Autodesk Inventor part; units mm, degrees
ref_plane "YZ Plane" through (0, 0, 0) normal (1, 0, 0) x (0, 1, 0)
ref_plane "XZ Plane" through (0, 0, 0) normal (0, 1, 0) x (-1, 0, 0)
ref_plane "XY Plane" through (0, 0, 0) normal (0, 0, 1) x (1, 0, 0)
sketch "스케치1" plane through (0, 0, 0) normal (0, 0, 1) x (1, 0, 0)
  line L0 (7.15, 10.1828) -> (7.15, 9)
  arc A0 (7.15, 9) -> (9.15, 7) centre (9.15, 9) ccw
  line L1 (9.15, 7) -> (11.2, 7)
  arc A1 (12.2, 6) -> (11.2, 7) centre (11.2, 6) ccw
  line L2 (12.2, 6) -> (12.2, -27)
  line L3 (-12.2, -27) -> (-12.2, 6)
  arc A2 (-11.2, 7) -> (-12.2, 6) centre (-11.2, 6) ccw
  line L4 (-11.2, 7) -> (-9.15, 7)
  arc A3 (-9.15, 7) -> (-7.15, 9) centre (-9.15, 9) ccw
  line L5 (-7.15, 9) -> (-7.15, 10.1828)
  spline S0 degree 3 poles (-7.15, 10.1828) (-7.15, 10.4656) (-7.1021, 10.8015) (-6.9309, 11.2744) (-6.801, 11.5043) (-6.5407, 11.7954) (-6.3826, 11.9196) (-6.2267, 12) knots -0.826314 -0.826314 -0.826314 -0.826314 -0.741468 -0.741468 -0.675447 -0.675447 -0.624321 -0.624321 -0.624321 -0.624321
  line L6 (-12.7, 12) -> (-6.2267, 12)
  line L7 (-17.8, 6) -> (-12.7, 12)
  line L8 (-17.8, -32.6) -> (-17.8, 6)
  line L9 (17.8, 6) -> (17.8, -32.6)
  line L10 (12.7, 12) -> (17.8, 6)
  line L11 (6.2267, 12) -> (12.7, 12)
  spline S1 degree 3 poles (6.2267, 12) (6.3826, 11.9196) (6.5407, 11.7954) (6.801, 11.5043) (6.9309, 11.2744) (7.1021, 10.8015) (7.15, 10.4656) (7.15, 10.1828) knots -0.510875 -0.510875 -0.510875 -0.510875 -0.459749 -0.459749 -0.393728 -0.393728 -0.308882 -0.308882 -0.308882 -0.308882
  circle A4 centre (15, 4.5) radius 1.35
  circle A5 centre (-15, 4.5) radius 1.35
  line L12 (-10.5, -74.2) -> (10.5, -74.2)
  line L13 (10.5, -73.725) -> (10.5, -68.6)
  line L14 (10.5, -68.6) -> (13, -68.6)
  line L15 (13, -68.6) -> (15, -68.6)
  line L16 (15, -74.6) -> (15, -68.6)
  line L17 (10.5, -74.6) -> (10.5, -73.725)
  line L18 (-10.5, -73.725) -> (-10.5, -68.6)
  line L19 (-10.5, -74.6) -> (-10.5, -73.725)
  line L20 (-10.5, -68.6) -> (-13, -68.6)
  line L21 (-13, -68.6) -> (-15, -68.6)
  line L22 (-15, -74.6) -> (-15, -68.6)
  line L23 (-16.75, -74.2) -> (-15, -74.2)
  line L24 (-12.6075, -38.4) -> (-12.6075, -53.4)
  line L25 (-12.6075, -53.4) -> (12.6075, -53.4)
  line L26 (12.6075, -53.4) -> (12.6075, -38.4)
  line L27 (-3.0413, -53.4) -> (2.9587, -53.4)
  line L28 (-3.0413, -53.4) -> (2.9587, -53.4)
  line L29 (-3.1413, -53.5) -> (3.0587, -53.5)
  line L30 (3.0587, -53.5) -> (3.0587, -47.3)
  line L31 (3.0587, -47.3) -> (-3.1413, -47.3)
  line L32 (-3.1413, -47.3) -> (-3.1413, -53.5)
  circle A6 centre (-3.1413, -47.3) radius 1
  circle A7 centre (-3.1413, -53.4) radius 1
  circle A8 centre (3.0587, -47.3) radius 1
  circle A9 centre (3.0587, -53.4) radius 1
  circle A10 centre (7.8038, -50.4) radius 1.25
  circle A11 centre (-7.8037, -50.4) radius 1.25
  line L33 (21, -65.4) -> (-21, -65.4)
  line L34 (-21, -65.4) -> (-21, -59.4)
  line L35 (-12.6075, -59.4) -> (-21, -59.4)
  line L36 (-12.6075, -59.4) -> (-12.6075, -47.4)
  line L37 (12.6075, -47.4) -> (-12.6075, -47.4)
  line L38 (12.6075, -59.4) -> (12.6075, -47.4)
  line L39 (21, -59.4) -> (12.6075, -59.4)
  line L40 (21, -65.4) -> (21, -59.4)
  line L41 (12.7, 12) -> (9.2, 12)
  line L42 (12.7, 12) -> (17.8, 6)
  line L43 (17.8, 6) -> (17.8, -32.6)
  line L44 (17.8, -32.6) -> (12.7, -38.6)
  line L45 (12.7, -38.6) -> (-12.7, -38.6)
  line L46 (-12.7, -38.6) -> (-17.8, -32.6)
  line L47 (-17.8, -32.6) -> (-17.8, 6)
  line L48 (-17.8, 6) -> (-12.7, 12)
  line L49 (-9.2, 12) -> (-12.7, 12)
  arc A12 (-9.2, 12) -> (-12.2, 9) centre (-9.2, 9) ccw
  line L50 (-12.2, -30) -> (-12.2, 9)
  arc A13 (-12.2, -30) -> (-9.2, -33) centre (-9.2, -30) ccw
  line L51 (9.2, -33) -> (-9.2, -33)
  arc A14 (9.2, -33) -> (12.2, -30) centre (9.2, -30) ccw
  line L52 (12.2, 9) -> (12.2, -30)
  arc A15 (12.2, 9) -> (9.2, 12) centre (9.2, 9) ccw
  circle A16 centre (15, 4.5) radius 1.35
  circle A17 centre (15, -12.5) radius 1.35
  circle A18 centre (8.5, -35.8) radius 1.35
  circle A19 centre (-15, 4.5) radius 1.35
  circle A20 centre (-15, -12.5) radius 1.35
  circle A21 centre (-8.5, -35.8) radius 1.35
  circle A22 centre (15, -29.5) radius 1.35
  circle A23 centre (-15, -29.5) radius 1.35
  line L53 (-12.7, 11.8) -> (-10.7492, 11.8)
  arc A24 (-10.7492, 11.8) -> (-12.4, 9) centre (-9.2, 9) ccw
  line L54 (-12.4, 9) -> (-12.4, -30)
  arc A25 (-12.4, -30) -> (-9.2, -33.2) centre (-9.2, -30) ccw
  line L55 (-9.2, -33.2) -> (9.2, -33.2)
  arc A26 (9.2, -33.2) -> (12.4, -30) centre (9.2, -30) ccw
  line L56 (12.4, -30) -> (12.4, 9)
  arc A27 (12.4, 9) -> (10.7492, 11.8) centre (9.2, 9) ccw
  line L57 (10.7492, 11.8) -> (12.7, 11.8)
  line L58 (-17.6, -21) -> (-12.3919, -21)
  line L59 (-17.6, -21) -> (-17.8, -21)
  line L60 (17.5991, -21) -> (17.8, -21)
  line L61 (-12.3919, -21) -> (-12.2, -21)
  line L62 (12.4, -21) -> (12.2, -21)
  line L63 (12.4, -21) -> (17.5991, -21)
  point P0 (3.0587, -52.4)
  point P1 (4.0587, -53.4)
  point P2 (-4.1413, -53.4)
  point P3 (-3.1413, -52.4)
  point P4 (-3.1413, -48.3)
  point P5 (-2.1413, -47.3)
  point P6 (2.0587, -47.3)
  point P7 (3.0587, -48.3)
  point P8 (2.0637, -53.5)
  point P9 (2.0587, -53.4)
  point P10 (-2.1413, -53.4)
  point P11 (-2.1463, -53.5)
  point P12 (-2.1463, -47.4)
  point P13 (2.0637, -47.4)
  point P14 (12.6075, -38.6)
  point P15 (-12.4, -21)
  point P16 (-12.6075, -38.6)
  dimension "d6" = 15
  dimension "d8" = 2
  dimension "d9" = 2
  dimension "d10" = 2
  dimension "d11" = 2
  dimension "d43" = 0.2
extrude "돌출1" add sketch "스케치1" along normal blind 6 contours L9 L44 L45 L46 L8 L59 L58 L54 A25 L55 A26 L56 L63 L60 | L26 L37 A8 L31 A6 L24 L45 | L26 L25 A9 L30 A8 L37 | L37 A6 L32 A7 L25 L24 | L37 A6 L31 A8 | A10 | A11
sketch "스케치3" plane through (0, 0, 0) normal (0, 0, -1) x (-1, 0, 0)
  line L0 (3.1413, -52.4) -> (3.1413, -48.3)
  line L1 (12.6075, -38.6) -> (12.6075, -53.4)
  line L2 (7.8037, -50.4) -> (7.8037, -53.4)
  line L3 (12.6075, -53.4) -> (4.1413, -53.4)
  line L4 (7.8037, -50.4) -> (7.8037, -45.7034)
  line L5 (12.6075, -47.4) -> (-12.6075, -47.4)
  line L6 (-12.6075, -47.4) -> (-12.6075, -59.4)
  line L7 (-12.6075, -59.4) -> (12.6075, -59.4)
  line L8 (12.6075, -59.4) -> (12.6075, -47.4)
  line L9 (-12.6075, -53.4) -> (12.6075, -53.4)
  line L10 (4.1413, -53.4) -> (-12.6075, -53.4)
  line L11 (0, -53.4) -> (0, -47.4)
  circle A0 centre (10.2056, -50.4) radius 1.35
  circle A1 centre (5.4019, -50.4) radius 1.35
  circle A2 centre (-10.2056, -50.4) radius 1.35
  circle A3 centre (-5.4019, -50.4) radius 1.35
  point P0 (0, 0)
  point P1 (12.6075, -38.4)
  point P2 (-4.0587, -53.4)
  point P3 (-3.0587, -53.4)
extrude "돌출2" cut sketch "스케치3" against normal up to next contours A0 | A1 | A2 | A3
properties part number "arm_connect_5" material "PMMA 플라스틱"
Verification items for the finished model (mm, model axes). A direction names the side the tool comes from. Round coordinates to 2 decimals unless told otherwise and drop trailing zeros. Loops run counter-clockwise (first coordinate to the right, second up) from the corner with the lowest first, then second, coordinate; pieces in that order, holes last. Notation, with made-up numbers: (1.25, 1) - (13.25, 1) arc R18 cw to (13.25, 13) - close; hole circle Ø5 at (40, 63.25). An arc over 180 degrees is marked (long way). Use a Markdown table: item, result. Add a question column.
1. Release check for a two-part mould opening along X. For faces 1 (the face through (15.286, -35.558, 2.958)), 2 (the face through (3.059, -50, 3)), 3 (the face through (-12.608, -46, 3)) record: released by +X, released by -X, zero draft, split by the parting line, or undercut.
2. Gauge pin test, flat ends, axial feed: pin 1 (3.5 mm diameter, centred on x = -15, y = -29.5, fed in from +Z); pin 2 (1.2 mm diameter, centred on y = -49.5, z = 4, fed in from -X); pin 3 (3 mm diameter, centred on y = -35, z = 4, fed in from +X) (3 decimals); pin 4 (3 mm diameter, centred on x = -1.5, z = 2.5, fed in from +Y). Record the tip position at first contact, or that the pin passes through.
3. Section check A-A, the plane y = -29.5. Record the boundary of the cut face in (x, z), plus the area to 3 significant figures.
4. Access from +Z, -Z, +X, -X, +Y, -Y to the whole of each face (thin tool, end or side, straight path). Record for faces 4 (the face through (-12.4, -25, 3)), 5 (the face through (-5.11, -51.72, 2.96)), 6 (the face through (-3.856, -52.701, 2.958)).
5. Section check B-B, the plane y = -35.8. Record the boundary of the cut face in (x, z), plus the area to 3 significant figures.
6. Thickness scan on probe 1 along Y at (x, z) = (-8.5, 3.6); probe 2 along X at (y, z) = (-27, 5.5); probe 3 along Y at (x, z) = (9, 3.15). Record the ranges inside material, lowest first. Write a range as [from, to].
7. Section check D-D, the plane y = -50.4. Record the boundary of the cut face in (x, z).
8. Section check C-C, the plane x = 10.5. Record the boundary of the cut face in (y, z).
Checks:
| question | item | result |
|---|---|---|
| 1 | face 1 | released by +X |
| 1 | face 2 | undercut |
| 1 | face 3 | released by -X |
| 2 | pin 1 | stops at z = 6 |
| 2 | pin 2 | stops at x = -12.61 |
| 2 | pin 3 | stops at x = 17.035 |
| 2 | pin 4 | stops at y = -33.2 |
| 3 | outline | (-17.8, 0) - (-16.35, 0) - (-16.35, 6) - (-17.8, 6) - close; (-13.65, 0) - (-12.4, 0) - (-12.4, 6) - (-13.65, 6) - close; (12.4, 0) - (13.65, 0) - (13.65, 6) - (12.4, 6) - close; (16.35, 0) - (17.8, 0) - (17.8, 6) - (16.35, 6) - close |
| 3 | area | 32.4 mm^2 |
| 4 | face 4 | +Z, -Z, +Y |
| 4 | face 5 | +Z, -Z |
| 4 | face 6 | +Z, -Z, -Y |
| 5 | outline | (-15.08, 0) - (-9.85, 0) - (-9.85, 6) - (-15.08, 6) - close; (-7.15, 0) - (7.15, 0) - (7.15, 6) - (-7.15, 6) - close; (9.85, 0) - (15.08, 0) - (15.08, 6) - (9.85, 6) - close |
| 5 | area | 149 mm^2 |
| 6 | probe 1 | y = [-53.4, -37.15], [-34.45, -33.2] |
| 6 | probe 2 | x = [-17.8, -12.4], [12.4, 17.8] |
| 6 | probe 3 | y = [-53.4, -51.01], [-49.79, -37.05], [-34.55, -33.2] |
| 7 | outline | (-12.61, 0) - (-11.56, 0) - (-11.56, 6) - (-12.61, 6) - close; (-8.86, 0) - (-6.75, 0) - (-6.75, 6) - (-8.86, 6) - close; (-4.05, 0) - (-3.14, 0) - (-3.14, 6) - (-4.05, 6) - close; (3.06, 0) - (4.05, 0) - (4.05, 6) - (3.06, 6) - close; (6.75, 0) - (8.86, 0) - (8.86, 6) - (6.75, 6) - close; (11.56, 0) - (12.61, 0) - (12.61, 6) - (11.56, 6) - close |
| 8 | outline | (-53.4, 0) - (-51.72, 0) - (-51.72, 6) - (-53.4, 6) - close; (-49.08, 0) - (-32.92, 0) - (-32.92, 6) - (-49.08, 6) - close |
